```python
from build123d import *

# Parameters (mm, degrees)
SKETCH1_R          = 8.7376
SKETCH1_R_2        = 4.953
BASE_EXTRUDE_DEPTH = 2.3876
CUT_EXTRUDE1_DEPTH = 13.58538602


with BuildPart() as part:
    # Sketch1 → Base-Extrude (new body)
    with BuildSketch(Plane(origin=(0, 0, 0), x_dir=(1, 0, 0), z_dir=(0, 1, 0))):
        with Locations(Location((0, 0, 0), (0, 0, 270))):
            Circle(SKETCH1_R)
        with Locations(Location((0, 0, 0), (0, 0, 270))):
            Circle(SKETCH1_R_2, mode=Mode.SUBTRACT)
    extrude(amount=BASE_EXTRUDE_DEPTH)

    # Sketch2 → Cut-Extrude1 (cut, through all)
    with BuildSketch(Plane(origin=(0, 2.3876, 0), x_dir=(-1, 0, 0), z_dir=(0, 1, 0))):
        with BuildLine():
            Line((-8.729289362, -0.381), (0, -0.381))
            Line((0, -0.381), (0, 0.381))
            Line((0, 0.381), (-8.729289362, 0.381))
            ThreePointArc((-8.729289362, 0.381), (-8.7376, 0), (-8.729289362, -0.381))
        make_face()
    extrude(amount=-CUT_EXTRUDE1_DEPTH, mode=Mode.SUBTRACT)


solid = part.part
```
Can you work these out from the model? Positions are in its coordinate system, mm. A direction names the side the tool comes from. Round coordinates to 2 decimals unless told otherwise and drop trailing zeros. Loops run counter-clockwise (first coordinate to the right, second up) from the corner with the lowest first, then second, coordinate; pieces in that order, holes last. Notation, with made-up numbers: (46, 17.25) -> (105, 17.25) arc R27 ccw to (105, 35.25) -> close; hole circle Ø1 at (-35, 14.5). An arc over 180 degrees is marked (long way). One line per item, written item: value. Start each with the question number.
1. If we section it at D-D, the plane y = 1.95: Write out the boundary of the cut face in (x, z).
2. If we section it at A-A, the plane x = 1.5: Write out the boundary of the cut face in (y, z).
3. If we section it at C-C, the plane z = 0: Write out the boundary of the cut face in (x, y), then the cut area to 3 significant figures.
4. If we section it at B-B, the plane z = 3: Write out the boundary of the cut face in (x, y).
5. For faces 3 (the flat face through (-4, 2.388, 4)), 4 (the flat face through (7, 1, -0.381)), which set-ups out of +Z, -Z, +X, -X, +Y, -Y let a thin tool reach every point of the face, with its end or its side?
6. If we mould it in two halves opening along Z, with no side actions, what happens to faces 1 (the flat face through (-4, 0, 4)), 2 (the cylindrical face through (-4.95, 1.18, -0.21))? For each: pulls with the +Z half, pulls with the -Z half, needs draft (parallel to the pull), parting line crosses it, or undercut.
7. If I drill on probe 1 along Z at (x, y) = (0, 0.5); probe 2 along X at (y, z) = (0.2, -1.25); probe 3 along Z at (x, y) = (1.75, 0.3), over which ranges is the centre line in solid material (lowest first)?
8. For pin 1 (1.2 mm diameter, centred on x = 6.5, y = 1, fed in from -Z), with a flat end and sliding along its axis, tell me the tip position at first contact or that it passes through.
Calculated:
1. outline: (4.94, -0.38) arc R4.95 cw (long way) to (4.94, 0.38) -> (8.73, 0.38) arc R8.74 ccw (long way) to (8.73, -0.38) -> close
2. outline: (0, -8.61) -> (2.39, -8.61) -> (2.39, -4.72) -> (0, -4.72) -> close; (0, 4.72) -> (2.39, 4.72) -> (2.39, 8.61) -> (0, 8.61) -> close
3. outline: (-8.74, 0) -> (-4.95, 0) -> (-4.95, 2.39) -> (-8.74, 2.39) -> close
3. area: 9.04 mm²
4. outline: (-8.21, 0) -> (-3.94, 0) -> (-3.94, 2.39) -> (-8.21, 2.39) -> close; (3.94, 0) -> (8.21, 0) -> (8.21, 2.39) -> (3.94, 2.39) -> close
5. face 3: +Z, -Z, +X, -X, +Y
5. face 4: +X, +Y, -Y
6. face 1: needs draft
6. face 2: undercut
7. probe 1: z = -8.74 to -4.95, 4.95 to 8.74
7. probe 2: x = -8.65 to -4.79, 4.79 to 8.65
7. probe 3: z = -8.56 to -4.63, 4.63 to 8.56
8. pin 1: stops at z = -6.44
